For this review, use the dimensioned drawing (mm, ordinates from the lowest corner) and the shaded views. Coordinates: 2 decimals unless noted, no trailing zeros. Write each loop counter-clockwise with the first axis right and the second up, starting at its lowest first coordinate (ties: lowest second). Pieces come first, ordered by that corner, then holes. Notation, with made-up numbers: M 61,42.5 L 120,42.5 A23 cw 120,59.5 Z; hole C 52.5,74 d3. An arc over 180 degrees is marked long. Return JSON: item names as keys, results as strings. Group by question number.
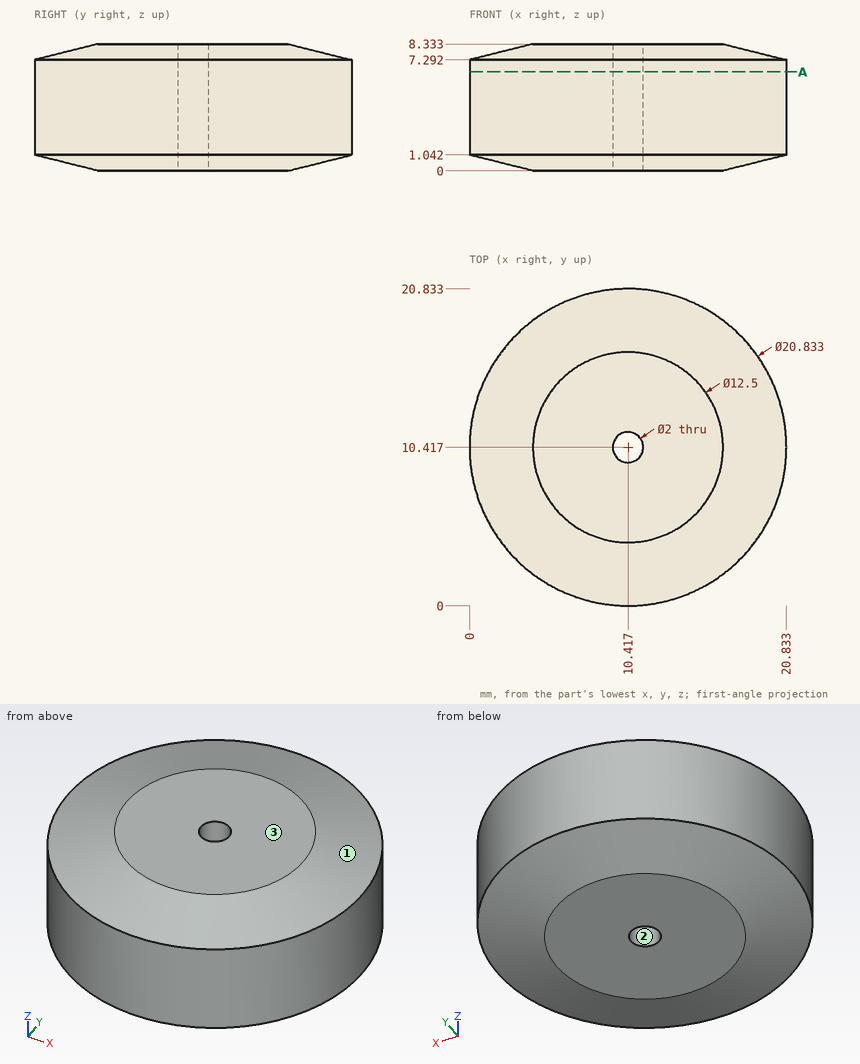
Item 1: The part is to be moulded in two halves that separate along Y. For the marked faces 1, 2 and 3, say which applies: pulls with the +Y half, pulls with the -Y half, needs draft (parallel to the pull), parting line crosses it, or undercut.
Item 2: Add section A-A (z = 6.5). Write out the cut boundary in (x, y), plus the area to 3 significant figures.
Item 3: For line 1 (Y direction, x = 10, z = 2) (1 decimal); line 2 (Y direction, x = 11, z = 5.25) (1 decimal); line 3 (Y direction, x = 7.5, z = 2), list the stretches that pass through material, from the lowest coordinate up.
Item 4: For pin 1 (1.8 mm diameter, centred on x = 10.42, y = 10.42, fed in from +Z); pin 2 (1 mm diameter, centred on x = 3, y = 12, fed in from +Z) (1 decimal), all flat-tipped, find the tip position at first contact; note any pin that passes through.
Geometry check:
{
 "1": {"face 1": "parting line crosses it", "face 2": "undercut", "face 3": "needs draft"},
 "2": {"outline": "C 10.42,10.42 d20.83; hole C 10.42,10.42 d2", "area": "338 mm^2"},
 "3": {"line 1": "0 to 9.5, 11.3 to 20.8", "line 2": "0 to 9.6, 11.2 to 20.8", "line 3": "0.42 to 20.42"},
 "4": {"pin 1": "through", "pin 2": "z = 8.1"}
}
